```python
from build123d import *

# Parameters (mm, degrees)
F0_W     = 75
F0_H     = 50
F0_R     = 6
F1_DEPTH = 10
F2_W     = 25
F2_H     = 50
F3_DEPTH = 30
F5_DEPTH = 40.001
F6_R     = 5
F7_R     = 4.99999


# Not quite as in the source:
# - a fillet or chamfer is up to 0.001 mm smaller than in the source, because OpenCascade refuses the exact size


with BuildPart() as f1:
    # F0 (on Front) → F1 (new body)
    with BuildSketch(Plane.XZ):
        with Locations((-12.5, 0)):
            Rectangle(F0_W, F0_H)
        with Locations((-35.368822515, -14)):
            Circle(F0_R, mode=Mode.SUBTRACT)
        with Locations((-14, 0)):
            Circle(F0_R, mode=Mode.SUBTRACT)
        with Locations((-34, 14)):
            Circle(F0_R, mode=Mode.SUBTRACT)
    extrude(amount=F1_DEPTH)

    # F2 (on face) → F3 (join)
    with BuildSketch(Plane.XZ.offset(10)):
        with Locations((12.5, 0)):
            Rectangle(F2_W, F2_H)
    extrude(amount=F3_DEPTH)

    # F4 (on face) → F5 (cut, through all)
    with BuildSketch(Plane.XZ.offset(40)):
        Polygon((25, -4.6425589255), (25, 6.4739544771), (15, 12.247457169), (15, -10.4160616174), align=None)
    extrude(amount=-F5_DEPTH, mode=Mode.SUBTRACT)

    # F6
    f6_edges = [f1.edges().sort_by_distance(p)[0] for p in [
        (-50, -5, -25),
        (-50, -5, 25),
        (0, -10, 0),
    ]]
    fillet(f6_edges, radius=F6_R)

    # F7 (radius 5 in the source; OpenCascade refuses exactly that, so slightly less here)
    f7_edges = [f1.edges().sort_by_distance(p)[0] for p in [
        (-25, -10, -25),
        (12.5, -40, -25),
        (0, -40, 0),
        (12.5, -40, 25),
    ]]
    fillet(f7_edges, radius=F7_R)


solid = f1.part
```
Design review of the part built by this model. Coordinates are the model's own, in mm. A direction names the side the tool comes from. Coordinates: 2 decimals unless noted, no trailing zeros. Write each loop counter-clockwise with the first axis right and the second up, starting at its lowest first coordinate (ties: lowest second). Pieces come first, ordered by that corner, then holes.
1) To check wall thickness, follow L1, parallel to Z at x = -34, y = -5.5; L2, parallel to Z at x = -34, y = -7.5; L3, parallel to X at y = -23, z = -14. State the ranges of each line that lie inside material, in increasing order.
2) Add section B-B (x = -14). Write out the cut boundary in (y, z), plus the area to 3 significant figures.
3) Mouldability with a two-part tool opening along Z and no side actions: class faces 1 (the cylindrical face through (-32.143, -4.93, -8.941)), 2 (the flat face through (5, -13, -25)), 3 (the flat face through (25, -20, 16)), 4 (the cylindrical face through (-48, -3, 24)) as +Z half, -Z half, draft (parallel to the pull), parting line (faces both ways), or undercut.
4) Insertion check: pin 1 (8 mm diameter, centred on x = -9.5, z = -7, fed in from +Y); pin 2 (16 mm diameter, centred on y = -22.5, z = -2, fed in from -X); pin 3 (20 mm diameter, centred on x = -33.5, z = -4.5, fed in from -Y); pin 4 (1.5 mm diameter, centred on x = -0.5, y = -9.5, fed in from +Z). Each pin has a flat end and moves straight along its axis. Give the tip position at first contact, or say it passes through.
5) Add section C-C (y = -24). Write out the cut boundary in (x, z), plus the area to 3 significant figures.
6) Machinability: for faces 5 (the cylindrical face through (2, -25, 24)), 6 (the cylindrical face through (-25, -8, -24)), 7 (the flat face through (-25, -10, 0)), which of the approach directions +Z, -Z, +X, -X, +Y, -Y give a long, thin tool a straight path to every point of the face, cutting with its end or side? Answer none if there is none.
7) Add section D-D (x = -43.5). Write out the cut boundary in (y, z), plus the area to 3 significant figures.
8) Add section A-A (z = 14). Write out the cut boundary in (x, y), plus the area to 3 significant figures.
Check result:
1. L1: z = -24.97 to -19.84, -8.16 to 8, 20 to 24.97
1. L2: z = -24.33 to -19.84, -8.16 to 8, 20 to 24.33
1. L3: x = 0 to 25
2. outline: (-10, -20) arc R5 ccw to (-5, -25) - (0, -25) - (0, -6) - (-10, -6) - close; (-10, 6) - (0, 6) - (0, 25) - (-5, 25) arc R5 ccw to (-10, 20) - close
2. area: 369 mm2
3. face 1: undercut
3. face 2: -Z half
3. face 3: draft
3. face 4: +Z half
4. pin 1: stops at y = 0
4. pin 2: stops at x = -0.03
4. pin 3: stops at y = -10
4. pin 4: stops at z = 24.52
5. outline: (0, -20) arc R5 ccw to (5, -25) - (25, -25) - (25, -4.64) - (15, -10.42) - (15, 12.25) - (25, 6.47) - (25, 25) - (5, 25) arc R5 ccw to (0, 20) - close
5. area: 1,070 mm2
6. face 5: +Z, -X, -Y
6. face 6: -Z, -X, -Y
6. face 7: +Z, -Z, -X, -Y
7. outline: (-10, -20) arc R5 ccw to (-5, -25) - (0, -25) - (0, 25) - (-5, 25) arc R5 ccw to (-10, 20) - close
7. area: 489 mm2
8. outline: (-50, -5) arc R5 ccw to (-45, -10) - (-40, -10) - (-40, 0) - (-50, 0) - close; (-28, -10) - (-5, -10) arc R5 cw to (0, -15) - (0, -35) arc R5 ccw to (5, -40) - (25, -40) - (25, 0) - (-28, 0) - close
8. area: 1,370 mm2
